Geometry: final body of the model. Coordinates: model frame, mm. Face numbers are marked on the shaded views. Give positions to 0.01 mm unless a question says otherwise; leave off trailing zeros. Order: outer loops, then holes, each group sorted by start corner. A loop starts at its lowest first (then second) coordinate and runs counter-clockwise, first axis right, second up. Notation, with made-up numbers: (-21, -26.75) - (13, -26.75) arc R32 ccw to (13, 8.25) - close; hole circle Ø9 at (80, 40.25). An arc over 180 degrees is marked (long way). Use one line per item in the form item = value.
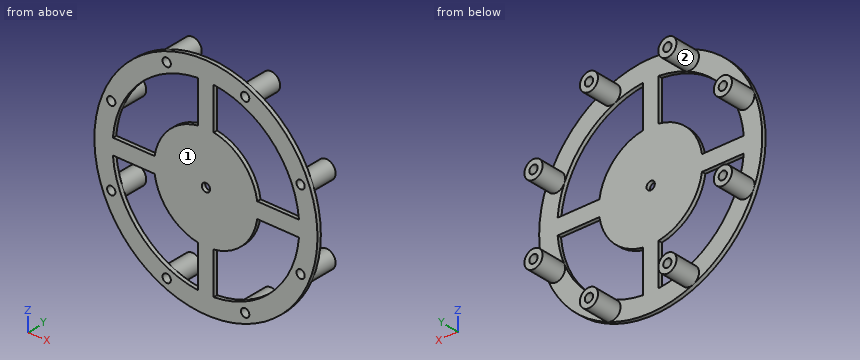
from build123d import *

# Parameters (mm, degrees)
ESBO_O1_R                = 43
ESBO_O1_R_2              = 1.6
RESSALTO_EXTRUS_O1_DEPTH = 0.75
ESBO_O2_R                = 3.5
ESBO_O2_R_2              = 1.6
RESSALTO_EXTRUS_O3_DEPTH = 10


with BuildPart() as part:
    # Esboço1 → Ressalto-extrusão1 (new, symmetric)
    with BuildSketch(Plane(origin=(0, 0, 0), x_dir=(1, 0, 0), z_dir=(0, 1, 0))):
        with Locations(Location((0, 0, 0), (0, 0, 270))):
            Circle(ESBO_O1_R)
        with Locations(Location((-36.493241534, 15.115995578, 0), (0, 0, 270))):
            Circle(ESBO_O1_R_2, mode=Mode.SUBTRACT)
        with Locations(Location((-15.115995578, 36.493241534, 0), (0, 0, 270))):
            Circle(ESBO_O1_R_2, mode=Mode.SUBTRACT)
        with Locations(Location((15.115995578, 36.493241534, 0), (0, 0, 270))):
            Circle(ESBO_O1_R_2, mode=Mode.SUBTRACT)
        with Locations(Location((36.493241534, 15.115995578, 0), (0, 0, 270))):
            Circle(ESBO_O1_R_2, mode=Mode.SUBTRACT)
        with Locations(Location((36.493241534, -15.115995578, 0), (0, 0, 270))):
            Circle(ESBO_O1_R_2, mode=Mode.SUBTRACT)
        with Locations(Location((15.115995578, -36.493241534, 0), (0, 0, 270))):
            Circle(ESBO_O1_R_2, mode=Mode.SUBTRACT)
        with Locations(Location((-15.115995578, -36.493241534, 0), (0, 0, 270))):
            Circle(ESBO_O1_R_2, mode=Mode.SUBTRACT)
        with Locations(Location((-36.493241534, -15.115995578, 0), (0, 0, 270))):
            Circle(ESBO_O1_R_2, mode=Mode.SUBTRACT)
        with Locations(Location((0, 0, 0), (0, 0, 270))):
            Circle(ESBO_O1_R_2, mode=Mode.SUBTRACT)
        with BuildLine():
            Line((-3, 19.773719933), (-3, 35.874782229))
            ThreePointArc((-3, 35.874782229), (-25.455844123, 25.455844123), (-35.874782229, 3))
            Line((-35.874782229, 3), (-19.773719933, 3))
            ThreePointArc((-19.773719933, 3), (-14.142135624, 14.142135624), (-3, 19.773719933))
        make_face(mode=Mode.SUBTRACT)
        with BuildLine():
            Line((3, 19.773719933), (3, 35.874782229))
            ThreePointArc((3, 35.874782229), (25.455844123, 25.455844123), (35.874782229, 3))
            Line((35.874782229, 3), (19.773719933, 3))
            ThreePointArc((19.773719933, 3), (14.142135624, 14.142135624), (3, 19.773719933))
        make_face(mode=Mode.SUBTRACT)
        with BuildLine():
            Line((19.773719933, -3), (35.874782229, -3))
            ThreePointArc((35.874782229, -3), (25.455844123, -25.455844123), (3, -35.874782229))
            Line((3, -35.874782229), (3, -19.773719933))
            ThreePointArc((3, -19.773719933), (14.142135624, -14.142135624), (19.773719933, -3))
        make_face(mode=Mode.SUBTRACT)
        with BuildLine():
            Line((-3, -19.773719933), (-3, -35.874782229))
            ThreePointArc((-3, -35.874782229), (-25.455844123, -25.455844123), (-35.874782229, -3))
            Line((-35.874782229, -3), (-19.773719933, -3))
            ThreePointArc((-19.773719933, -3), (-14.142135624, -14.142135624), (-3, -19.773719933))
        make_face(mode=Mode.SUBTRACT)
    extrude(amount=RESSALTO_EXTRUS_O1_DEPTH, both=True)

    # Esboço2 → Ressalto-extrusão3 (add)
    # profile 1 of 8: a face of its own
    with BuildSketch(Plane(origin=(0, 0.75, 0), x_dir=(1, 0, 0), z_dir=(0, 1, 0))):
        with Locations(Location((-15.115995578, 36.493241534, 0), (0, 0, 112.5))):
            Circle(ESBO_O2_R)
        with Locations(Location((-15.115995578, 36.493241534, 0), (0, 0, 270))):
            Circle(ESBO_O2_R_2, mode=Mode.SUBTRACT)
    # profile 2 of 8: a face of its own
    with BuildSketch(Plane(origin=(0, 0.75, 0), x_dir=(1, 0, 0), z_dir=(0, 1, 0))):
        with Locations(Location((15.115995578, 36.493241534, 0), (0, 0, 67.5))):
            Circle(ESBO_O2_R)
        with Locations(Location((15.115995578, 36.493241534, 0), (0, 0, 270))):
            Circle(ESBO_O2_R_2, mode=Mode.SUBTRACT)
    # profile 3 of 8: a face of its own
    with BuildSketch(Plane(origin=(0, 0.75, 0), x_dir=(1, 0, 0), z_dir=(0, 1, 0))):
        with Locations(Location((36.493241534, 15.115995578, 0), (0, 0, 22.5))):
            Circle(ESBO_O2_R)
        with Locations(Location((36.493241534, 15.115995578, 0), (0, 0, 270))):
            Circle(ESBO_O2_R_2, mode=Mode.SUBTRACT)
    # profile 4 of 8: a face of its own
    with BuildSketch(Plane(origin=(0, 0.75, 0), x_dir=(1, 0, 0), z_dir=(0, 1, 0))):
        with Locations(Location((36.493241534, -15.115995578, 0), (0, 0, 157.5))):
            Circle(ESBO_O2_R)
        with Locations(Location((36.493241534, -15.115995578, 0), (0, 0, 270))):
            Circle(ESBO_O2_R_2, mode=Mode.SUBTRACT)
    # profile 5 of 8: a face of its own
    with BuildSketch(Plane(origin=(0, 0.75, 0), x_dir=(1, 0, 0), z_dir=(0, 1, 0))):
        with Locations(Location((15.115995578, -36.493241534, 0), (0, 0, 112.5))):
            Circle(ESBO_O2_R)
        with Locations(Location((15.115995578, -36.493241534, 0), (0, 0, 270))):
            Circle(ESBO_O2_R_2, mode=Mode.SUBTRACT)
    # profile 6 of 8: a face of its own
    with BuildSketch(Plane(origin=(0, 0.75, 0), x_dir=(1, 0, 0), z_dir=(0, 1, 0))):
        with Locations(Location((-15.115995578, -36.493241534, 0), (0, 0, 67.5))):
            Circle(ESBO_O2_R)
        with Locations(Location((-15.115995578, -36.493241534, 0), (0, 0, 270))):
            Circle(ESBO_O2_R_2, mode=Mode.SUBTRACT)
    # profile 7 of 8: a face of its own
    with BuildSketch(Plane(origin=(0, 0.75, 0), x_dir=(1, 0, 0), z_dir=(0, 1, 0))):
        with Locations(Location((-36.493241534, -15.115995578, 0), (0, 0, 22.5))):
            Circle(ESBO_O2_R)
        with Locations(Location((-36.493241534, -15.115995578, 0), (0, 0, 270))):
            Circle(ESBO_O2_R_2, mode=Mode.SUBTRACT)
    # profile 8 of 8: a face of its own
    with BuildSketch(Plane(origin=(0, 0.75, 0), x_dir=(1, 0, 0), z_dir=(0, 1, 0))):
        with Locations(Location((-36.493241534, 15.115995578, 0), (0, 0, 157.5))):
            Circle(ESBO_O2_R)
        with Locations(Location((-36.493241534, 15.115995578, 0), (0, 0, 270))):
            Circle(ESBO_O2_R_2, mode=Mode.SUBTRACT)
    extrude(amount=RESSALTO_EXTRUS_O3_DEPTH)


solid = part.part
(1) Cut plane A-A on z = 0. Output: boundary loops of the cut face in (x, y).
Computed values:
outline = (-43, -0.75) - (-1.6, -0.75) - (-1.6, 0.75) - (-43, 0.75) - close; (1.6, -0.75) - (43, -0.75) - (43, 0.75) - (1.6, 0.75) - close
(2) Ray query, line 1 along X through (y, z) = (-0.25, -23.5); line 2 along X through (y, z) = (5.75, 15.5); line 3 along X through (y, z) = (6, 14.5). Return the intervals inside material, ascending.
Computed values:
line_1 = -36.01 to -27.27, -3 to 3, 27.27 to 36.01
line_2 = -39.97 to -38.05, -34.94 to -33.01, 33.01 to 34.94, 38.05 to 39.97
line_3 = -39.94 to -37.97, -35.02 to -33.05, 33.05 to 35.02, 37.97 to 39.94
(3) Contact query for flat-ended pins moving along their axis: pin 1 Ø5 at (x, y) = (-12.5, 8) entering from -Z; pin 2 Ø1.2 at (y, z) = (0, 30.5) entering from +X; pin 3 Ø3 at (x, z) = (36.49, -15.12) entering from +Y; pin 4 Ø21 at (x, z) = (-27.5, 31.5) entering from +Y. Output: stop coordinate, or through.
Computed values:
pin_1 = -39.99
pin_2 = 30.9
pin_3 = through
pin_4 = 10.75
(4) Pull-direction query (X, two-part tool) for the marked faces 1 and 2; classes: released by +X, released by -X, zero draft, split by the parting line, or undercut.
Computed values:
face_1 = zero draft
face_2 = undercut
(5) Cut plane B-B on x = 0. Output: boundary loops of the cut face in (y, z), plus the area to 3 significant figures.
Computed values:
outline = (-0.75, -43) - (0.75, -43) - (0.75, -1.6) - (-0.75, -1.6) - close; (-0.75, 1.6) - (0.75, 1.6) - (0.75, 43) - (-0.75, 43) - close
area = 124 mm²
(6) Cut plane D-D on z = -9.5. Output: boundary loops of the cut face in (x, y), plus the area to 3 significant figures.
Computed values:
outline = (-41.94, -0.75) - (-34.72, -0.75) - (-34.72, 0.75) - (-41.94, 0.75) - close; (-17.6, -0.75) - (17.6, -0.75) - (17.6, 0.75) - (-17.6, 0.75) - close; (34.72, -0.75) - (41.94, -0.75) - (41.94, 0.75) - (34.72, 0.75) - close
area = 74.4 mm²
(7) Cut plane C-C on y = 4. Give the number of separate pieces and of enclosed holes in the cut face, plus the area to 3 significant figures.
Computed values:
separate_pieces = 8
enclosed_holes = 8
area = 244 mm²
